Answer from the drawing. Dimensions are ordinates in mm from the lowest x, y and z of the part. A direction names the side the tool comes from. Give positions to 0.01 mm unless a question says otherwise; leave off trailing zeros. Loops run counter-clockwise (first coordinate to the right, second up) from the corner with the lowest first, then second, coordinate; pieces in that order, holes last. Notation, with made-up numbers: M 52.25,49.5 L 104.25,49.5 A13 ccw 104.25,56.5 Z; hole C 74.25,23 d1. An arc over 180 degrees is marked long. Use a Markdown table: item, result.
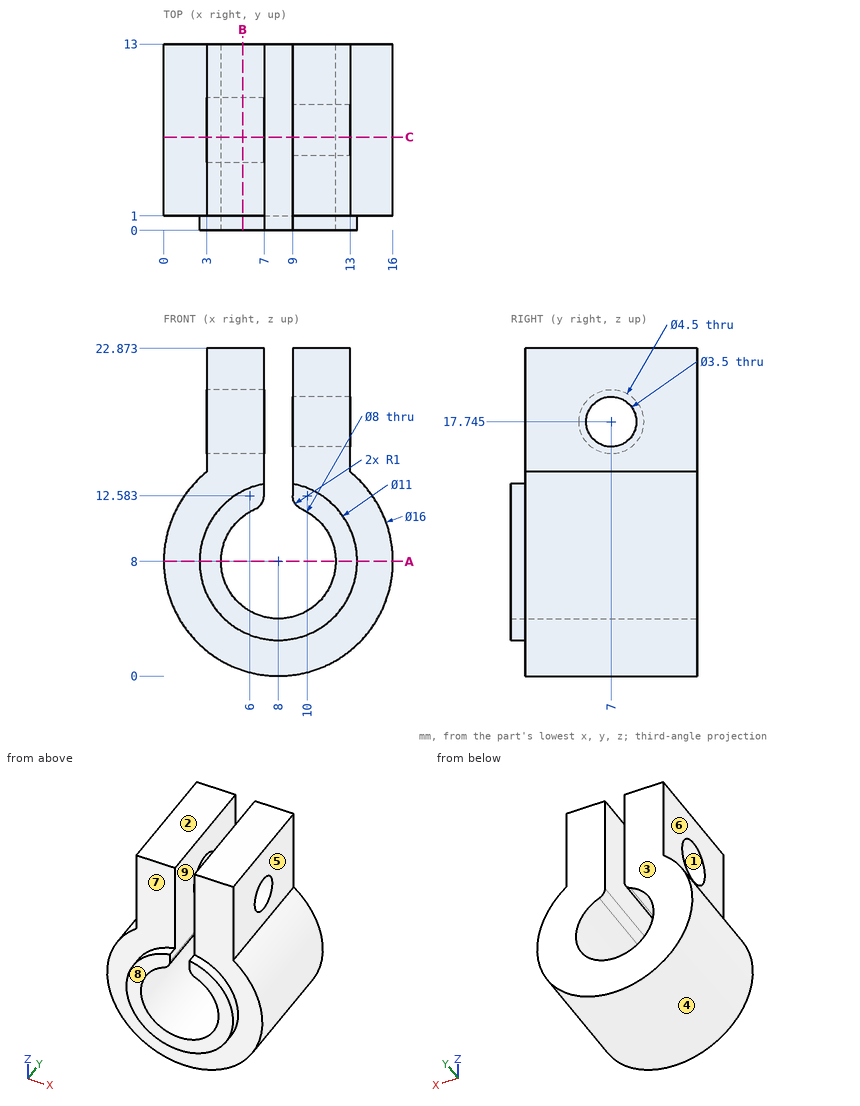
(1) Given P1, Ø4.5, axis at y = 10, z = 17.5, coming from the -X side; P2, Ø5, axis at y = 7, z = 17.74, coming from the +X side; P3, Ø2, axis at y = 5.5, z = 11, coming from the +X side, each flat-ended and moving along its own axis, determine where each tip first touches the part or whether it passes through.
Entries:
| item | result |
|---|---|
| P1 | stops at x = 3 |
| P2 | stops at x = 13 |
| P3 | stops at x = 15.75 |
(2) The mould has two halves that part along Z. Classify the marked faces 1, 2, 3 and 4: released by +Z, released by -Z, zero draft, split by the parting line, or undercut.
Entries:
| item | result |
|---|---|
| face 1 | undercut |
| face 2 | released by +Z |
| face 3 | zero draft |
| face 4 | split by the parting line |
(3) A cutting plane is placed at A-A (z = 8). Write down the section's boundary in (x, y).
Entries:
| item | result |
|---|---|
| outline | M 0,1 L 2.5,1 L 2.5,0 L 4,0 L 4,13 L 0,13 Z; M 12,0 L 13.5,0 L 13.5,1 L 16,1 L 16,13 L 12,13 Z |
(4) A cutting plane is placed at C-C (y = 6.5). Write down the section's boundary in (x, z) (1 decimal), and give its area (3 significant figures).
Entries:
| item | result |
|---|---|
| outline | M 3,14.2 A8 ccw long 13,14.2 L 13,16.1 L 9,16.1 L 9,12.6 A1 ccw 9.6,11.7 A4 cw long 6.4,11.7 A1 ccw 7,12.6 L 7,15.6 L 3,15.6 Z; M 3,19.9 L 7,19.9 L 7,22.9 L 3,22.9 Z; M 9,19.4 L 13,19.4 L 13,22.9 L 9,22.9 Z |
| area | 172 mm² |
(5) Which of the six approach directions +Z, -Z, +X, -X, +Y, -Y give full straight-line access (tool end or side, diameter ignored) to the marked faces 5, 6, 7, 8 and 9?
Entries:
| item | result |
|---|---|
| face 5 | +Z, +X, +Y, -Y |
| face 6 | +Z, -X, +Y, -Y |
| face 7 | -Y |
| face 8 | +Z, -Z, +X, -X, -Y |
| face 9 | +Z, +Y, -Y |
(6) Consider probe 1 along X at (y, z) = (11, 18.5); probe 2 along X at (y, z) = (3.5, 8); probe 3 along Y at (x, z) = (3, 3.5). Determine where each line is inside the solid, lowest interval first. Write a range as [from, to].
Entries:
| item | result |
|---|---|
| probe 1 | x = [3, 7], [9, 13] |
| probe 2 | x = [0, 4], [12, 16] |
| probe 3 | y = [1, 13] |
(7) A cutting plane is placed at B-B (x = 5.5). Count the separate pieces of the cut face and the enclosed holes in it, and give its area (3 significant figures).
Entries:
| item | result |
|---|---|
| separate pieces | 2 |
| enclosed holes | 1 |
| area | 182 mm² |
